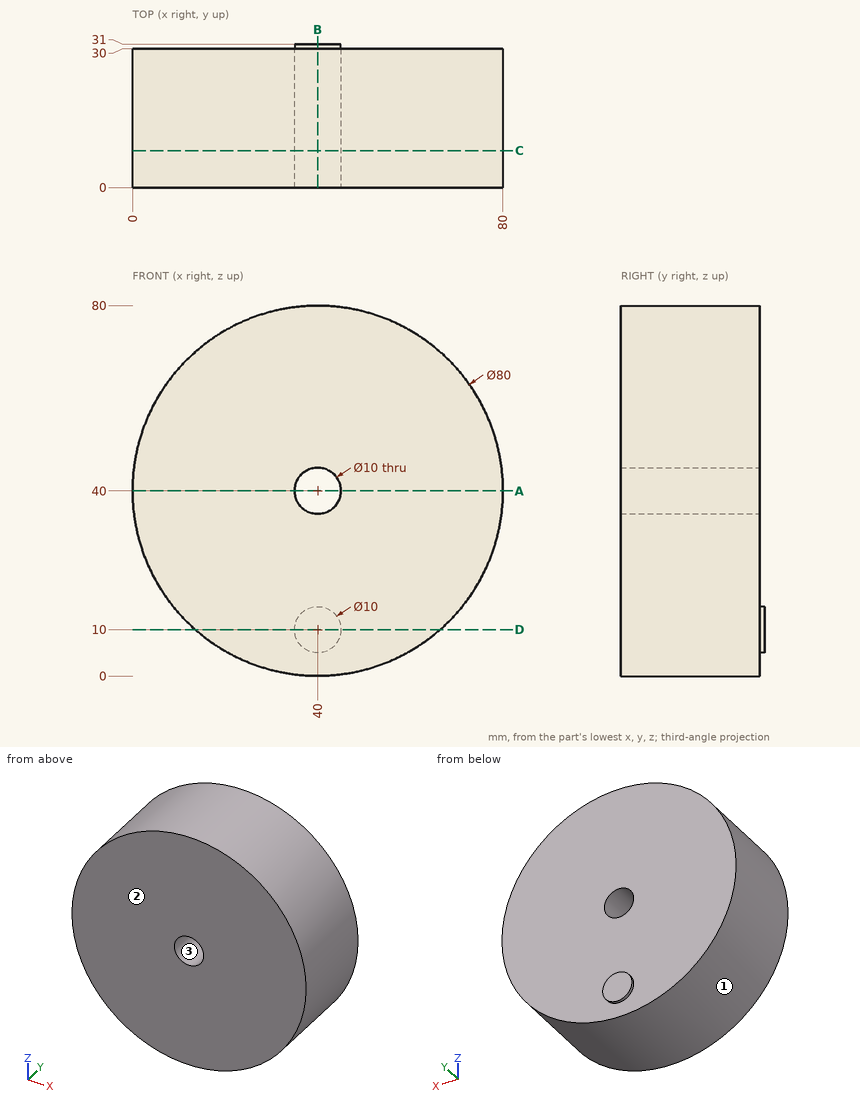
Could you check a few things on this drawing? It's one solid part, dimensions in mm from its lowest x, y, z. Round coordinates to 2 decimals unless told otherwise and drop trailing zeros. Write each loop counter-clockwise with the first axis right and the second up, starting at its lowest first coordinate (ties: lowest second). Pieces come first, ordered by that corner, then holes. Notation, with made-up numbers: (-9, -37.5) -> (1, -37.5) arc R20 ccw to (1, -5.5) -> close; hole circle Ø9 at (48, -36.5). An arc over 180 degrees is marked (long way). Use one line per item in the form item = value. Start each with the question number.
Q1. Imagine slicing it at A-A (z = 40). Please give me the cut outline in (x, y).
Q2. Imagine slicing it at D-D (z = 10). Please give me the cut outline in (x, y), then the cut area to 3 significant figures.
Q3. If I drill on probe 1 along Z at (x, y) = (40, 15.75); probe 2 along Y at (x, z) = (61, 36), over which ranges is the centre line in solid material (lowest first)? Write a range as [from, to].
Q4. Imagine slicing it at B-B (x = 40). Please give me the cut outline in (y, z).
Q5. I'm going to push flat-ended pins straight in: P1, Ø1.5, axis at x = 17.5, z = 63, coming from the +Y side; P2, Ø3, axis at y = 6, z = 12.5, coming from the -X side; P3, Ø8, axis at x = 26.5, y = 9.5, coming from the -Z side; P4, Ø8, axis at x = 40, z = 40, coming from the +Y side. Where does each tip first touch, or does it pass through?
Q6. We'd pull the mould along X, two halves only. Please class the marked faces 1, 2 and 3: +X half, -X half, draft (parallel to the pull), parting line (faces both ways), or undercut.
Q7. Imagine slicing it at C-C (y = 8). Please give me the cut outline in (x, z), then the cut area to 3 significant figures.
Worked out:
q1.outline = (0, 0) -> (35, 0) -> (35, 30) -> (0, 30) -> close; (45, 0) -> (80, 0) -> (80, 30) -> (45, 30) -> close
q2.outline = (13.54, 0) -> (66.46, 0) -> (66.46, 30) -> (45, 30) -> (45, 31) -> (35, 31) -> (35, 30) -> (13.54, 30) -> close
q2.area = 1,600 mm^2
q3.probe_1 = [0, 35], [45, 80]
q3.probe_2 = [0, 30]
q4.outline = (0, 0) -> (30, 0) -> (30, 5) -> (31, 5) -> (31, 15) -> (30, 15) -> (30, 35) -> (0, 35) -> close; (0, 45) -> (30, 45) -> (30, 80) -> (0, 80) -> close
q5.P1 = 30
q5.P2 = 9.6
q5.P3 = 1.14
q5.P4 = through
q6.face_1 = parting line
q6.face_2 = draft
q6.face_3 = undercut
q7.outline = circle Ø80 at (40, 40); hole circle Ø10 at (40, 40)
q7.area = 4,950 mm^2
